Autodesk Inventor part; units mm, degrees
ref_plane "YZ Plane" through (0, 0, 0) normal (1, 0, 0) x (0, 1, 0)
ref_plane "XZ Plane" through (0, 0, 0) normal (0, 1, 0) x (-1, 0, 0)
ref_plane "XY Plane" through (0, 0, 0) normal (0, 0, 1) x (1, 0, 0)
sketch "草图1" plane through (0, 0, 0) normal (1, 0, 0) x (0, 1, 0)
  circle A0 centre (0, 0) radius 1
  dimension "直径" = 2
extrude "拉伸1" add sketch "草图1" along normal blind 20
sketch "草图3" plane through (0, 0, 0) normal (0, 1, 0) x (-1, 0, 0)
  line L0 (-20, 1) -> (-20, -1)
  line L1 (0, -1) -> (0, 1)
  line L2 (0, 1) -> (-20, 1)
  line L3 (0, -1) -> (-20, -1)
  line L4 (-3, 1) -> (-3, -1)
  line L5 (0, 0.5) -> (-3, 0.5)
  line L6 (0, -0.5) -> (-3, -0.5)
  line L7 (-3, 0) -> (0, 0) construction
  dimension "长" = 3
  dimension "距离" = 1
extrude "拉伸2" cut sketch "草图3" along normal mid plane 10 contours L2 L1 L5 L4 | L4 L6 L1 L3
sketch "草图4" plane through (0, 0, 0) normal (0, 0, 1) x (1, 0, 0)
  line L0 (0, 1) -> (20, 1)
  line L1 (0, -1) -> (20, -1)
  line L2 (0, 0.866) -> (0, -0.866)
  line L3 (0, 0) -> (1.5, 0)
  circle A0 centre (1.5, 0) radius 0.5
  dimension "孔位置1" = 1.5
  dimension "孔径" = 1
extrude "拉伸3" cut sketch "草图4" along normal mid plane 10
properties part number "连接销1" material "木材(桦木)"
Source: CAD feature listing. Evaluate the final solid. Frame: model axes, mm. A direction names the side the tool comes from. Coordinates: 2 decimals unless noted, no trailing zeros. Order: outer loops, then holes, each group sorted by start corner. A loop starts at its lowest first (then second) coordinate and runs counter-clockwise, first axis right, second up. Notation, with made-up numbers: M 10,36.25 L 65,36.25 A21 cw 65,75.25 Z; hole C 77,-40 d3. An arc over 180 degrees is marked long. Write each question's results on one line, items separated by ' | '. Start each with the question number.
1) Line query: line 1 (X direction, y = 0, z = 0.1); line 2 (Y direction, x = 1.5, z = 0); line 3 (X direction, y = 0, z = 0.55). Output: solid intervals per line, ascending. Write a range as from..to.
2) Section query C-C (z = 0). Return the cut outline in (x, y).
3) Contact query for flat-ended pins moving along their axis: pin 1 Ø0.5 at (x, y) = (1.5, 0) entering from -Z; pin 2 Ø0.9 at (x, y) = (1.5, -0.5) entering from +Z; pin 3 Ø0.6 at (y, z) = (0, -0.5) entering from -X. Output: stop coordinate, or through.
4) Section query B-B (x = 1.5). Return the cut outline in (y, z), plus the area to 3 significant figures.
5) Access query for faces 1 (the face through (1.1, -0.6, -0.5)), 2 (the face through (0, 0, 0)), 3 (the face through (1.1, -0.6, 0.5)). Directions: +Z, -Z, +X, -X, +Y, -Y. A direction counts if a zero-diameter tool reaches every point of the face in a straight line with its end or side. Return the directions, or none.
6) Section query D-D (x = 13). Return the cut outline in (y, z), plus the area to 3 significant figures.
7) Section query A-A (y = 0). Return the cut outline in (x, z).
Answers:
1) line 1: x = 0..1, 2..20 | line 2: y = -1..-0.5, 0.5..1 | line 3: x = 3..20
2) outline: M 0,-1 L 20,-1 L 20,1 L 0,1 Z; hole C 1.5,0 d1
3) pin 1: passes through | pin 2: stops at z = 0.5 | pin 3: stops at x = 0
4) outline: M -0.87,-0.5 L -0.5,-0.5 L -0.5,0.5 L -0.87,0.5 A1 ccw Z; M 0.5,-0.5 L 0.87,-0.5 A1 ccw 0.87,0.5 L 0.5,0.5 Z | area: 0.913 mm^2
5) face 1: -Z, -X, +Y, -Y | face 2: +Z, -Z, -X, +Y, -Y | face 3: +Z, -X, +Y, -Y
6) outline: C 0,0 d2 | area: 3.14 mm^2
7) outline: M 0,-0.5 L 1,-0.5 L 1,0.5 L 0,0.5 Z; M 2,-0.5 L 3,-0.5 L 3,-1 L 20,-1 L 20,1 L 3,1 L 3,0.5 L 2,0.5 Z
